Read the model definition and answer for the solid it produces. Units are mm, in the model's axes. A direction names the side the tool comes from. Round coordinates to 2 decimals unless told otherwise and drop trailing zeros. Order: outer loops, then holes, each group sorted by start corner. A loop starts at its lowest first (then second) coordinate and runs counter-clockwise, first axis right, second up. Notation, with made-up numbers: M 87.25,-17 L 119.25,-17 A23 ccw 119.25,14 Z; hole C 24,46 d3. An arc over 180 degrees is marked long. Answer as CSV lines item,"result".
```python
from build123d import *

# Parameters (mm, degrees)
SKETCH004_W     = 40
SKETCH004_H     = 40
PAD001_DEPTH    = 40
SKETCH005_W     = 38.216385
SKETCH005_H     = 40.583008
POCKET002_DEPTH = 11.7
SKETCH006_R     = 1.75
POCKET003_DEPTH = 40.001
SKETCH007_W     = 20
SKETCH007_H     = 28
POCKET004_DEPTH = 35
SKETCH009_R     = 11
POCKET005_DEPTH = 28
SKETCH011_R     = 2.75
POCKET006_DEPTH = 36
SKETCH012_R     = 1.9
POCKET007_DEPTH = 7
CHAMFER003_SIZE = 0.9
SKETCH020_R     = 4.692288
POCKET013_DEPTH = 40.001
FILLET_R        = 3
SKETCH021_W     = 5
SKETCH021_H     = 10
POCKET014_DEPTH = 9
SKETCH022_W     = 5
SKETCH022_H     = 10
POCKET015_DEPTH = 12
SKETCH023_W     = 20
SKETCH023_H     = 14.49538
POCKET016_DEPTH = 20
CHAMFER006_SIZE = 3
CHAMFER007_SIZE = 2
FILLET001_R     = 1


with BuildPart() as part:
    # Sketch004 → Pad001 (new body)
    with BuildSketch(Plane.XY):
        Rectangle(SKETCH004_W, SKETCH004_H)
    extrude(amount=PAD001_DEPTH)

    # Sketch005 (on Face5 of Pad001) → Pocket002 (cut)
    with BuildSketch(Plane(origin=(0, 0, 0), x_dir=(1, 0, 0), z_dir=(0, 0, -1))):
        with Locations((-19.108192, -20.291504)):
            Rectangle(SKETCH005_W, SKETCH005_H)
    extrude(amount=-POCKET002_DEPTH, mode=Mode.SUBTRACT)

    # Sketch006 (on Face4 of Pocket002) → Pocket003 (cut, through all)
    with BuildSketch(Plane(origin=(0, 0, 0), x_dir=(1, 0, 0), z_dir=(0, 0, -1))):
        with Locations((-15.5, 15.5)):
            Circle(SKETCH006_R)
        with Locations((15.5, 15.5)):
            Circle(SKETCH006_R)
        with Locations((-15.5, -15.5)):
            Circle(SKETCH006_R)
        with Locations((15.5, -15.5)):
            Circle(SKETCH006_R)
    extrude(amount=-POCKET003_DEPTH, mode=Mode.SUBTRACT)

    # Sketch007 (on Face1 of Pocket003) → Pocket004 (cut)
    with BuildSketch(Plane(origin=(0, 20, 0), x_dir=(-1, 0, 0), z_dir=(0, 1, 0))):
        with Locations((0, 24)):
            Rectangle(SKETCH007_W, SKETCH007_H)
    extrude(amount=-POCKET004_DEPTH, mode=Mode.SUBTRACT)

    # Sketch009 (on Face9 of Pocket004) → Pocket005 (cut)
    with BuildSketch(Plane.XY.offset(40)):
        Circle(SKETCH009_R)
    extrude(amount=-POCKET005_DEPTH, mode=Mode.SUBTRACT)

    # Sketch011 (on Face9 of Pocket005) → Pocket006 (cut)
    with BuildSketch(Plane.XY.offset(40)):
        with Locations((-15.5, -15.5)):
            Circle(SKETCH011_R)
        with Locations((-15.5, 15.5)):
            Circle(SKETCH011_R)
        with Locations((15.5, 15.5)):
            Circle(SKETCH011_R)
        with Locations((15.5, -15.5)):
            Circle(SKETCH011_R)
    extrude(amount=-POCKET006_DEPTH, mode=Mode.SUBTRACT)

    # Sketch012 (on Face9 of Pocket006) → Pocket007 (cut)
    with BuildSketch(Plane.XY.offset(40)):
        with Locations((0, 15.5)):
            Circle(SKETCH012_R)
        with Locations((15.5, 0)):
            Circle(SKETCH012_R)
        with Locations((0, -15.5)):
            Circle(SKETCH012_R)
        with Locations((-15.5, 0)):
            Circle(SKETCH012_R)
    extrude(amount=-POCKET007_DEPTH, mode=Mode.SUBTRACT)

    # Chamfer003
    chamfer003_edges = [part.edges().sort_by_distance(p)[0] for p in [
        (10.747093, 2.345208, 12),
        (0, -11, 38),
        (10.747093, -2.345208, 12),
    ]]
    chamfer(chamfer003_edges, length=CHAMFER003_SIZE)

    # Sketch020 (on Face19 of Chamfer003) → Pocket013 (cut, through all)
    with BuildSketch(Plane(origin=(0, 0, 0), x_dir=(1, 0, 0), z_dir=(0, 0, -1))):
        Circle(SKETCH020_R)
    extrude(amount=-POCKET013_DEPTH, mode=Mode.SUBTRACT)

    # Fillet
    fillet_edges = [part.edges().sort_by_distance(p)[0] for p in [
        (-4.692288, 0, 5),
        (0, 4.692288, 5),
    ]]
    fillet(fillet_edges, radius=FILLET_R)

    # Sketch021 (on Face22 of Fillet) → Pocket014 (cut)
    with BuildSketch(Plane.YZ.offset(20)):
        with Locations((0, 31)):
            Rectangle(SKETCH021_W, SKETCH021_H)
    extrude(amount=-POCKET014_DEPTH, mode=Mode.SUBTRACT)

    # Sketch022 → Pocket015 (cut)
    with BuildSketch(Plane.XZ.offset(20)):
        with Locations((0, 31)):
            Rectangle(SKETCH022_W, SKETCH022_H)
    extrude(amount=-POCKET015_DEPTH, mode=Mode.SUBTRACT)

    # Sketch023 (on Face13 of Pocket015) → Pocket016 (cut)
    with BuildSketch(Plane(origin=(-20, 0, 0), x_dir=(0, -1, 0), z_dir=(-1, 0, 0))):
        with Locations((0, 40.24769)):
            Rectangle(SKETCH023_W, SKETCH023_H)
    extrude(amount=-POCKET016_DEPTH, mode=Mode.SUBTRACT)

    # Chamfer006
    chamfer006_edges = [part.edges().sort_by_distance(p)[0] for p in [
        (0, -20, 26),
        (20, 0, 26),
    ]]
    chamfer(chamfer006_edges, length=CHAMFER006_SIZE)

    # Chamfer007
    chamfer007_edges = [part.edges().sort_by_distance(p)[0] for p in [
        (-20, -20, 20),
        (-20, 20, 25.85),
        (20, -20, 20),
        (20, 20, 20),
    ]]
    chamfer(chamfer007_edges, length=CHAMFER007_SIZE)

    # Fillet001
    fillet001_edges = [part.edges().sort_by_distance(p)[0] for p in [
        (-2.5, -20, 31),
        (2.5, -20, 31),
        (20, -2.5, 31),
        (20, 2.5, 31),
    ]]
    fillet(fillet001_edges, radius=FILLET001_R)


solid = part.part
```
Item 1: A tool of negligible diameter and unlimited length cuts with its end or side. For faces 4 (the face through (0, -15, 24)), 5 (the face through (-5.41, -0.51, 4.93)), 6 (the face through (-15, 0, 33)), 7 (the face through (15, 2.5, 31)), 8 (the face through (15.142, 18.227, 22.252)), from which of +Z, -Z, +X, -X, +Y, -Y can it reach the whole face along a straight path? Write none if from no direction.
Ans:
face 4,"+Y"
face 5,"+Z, -Z, +Y"
face 6,"+Z, -X"
face 7,"+X"
face 8,"+Z"
Item 2: Find the intervals of material crossed by probe 1 along Z at (x, y) = (3, -12); probe 2 along X at (y, z) = (-11, 28.5); probe 3 along Y at (x, z) = (15.5, 32), in increasing order. Write a range as [from, to].
Ans:
probe 1,"[0, 10], [38, 40]"
probe 2,"[-20, -10], [10, 20]"
probe 3,"[-20, -18.25], [-12.75, -2.5], [2.5, 12.75], [18.25, 20]"
Item 3: A cutting plane is placed at C-C, the plane y = 15.5. Determine the outline of the cut face in (x, z).
Ans:
outline,"M -20,11.7 L -18.25,11.7 L -18.25,40 L -20,40 Z; M -12.75,11.7 L -10,11.7 L -10,38 L -1.9,38 L -1.9,40 L -12.75,40 Z; M 0,0 L 13.75,0 L 13.75,4 L 12.75,4 L 12.75,40 L 1.9,40 L 1.9,38 L 10,38 L 10,10 L 0,10 Z; M 17.25,0 L 20,0 L 20,40 L 18.25,40 L 18.25,4 L 17.25,4 Z"
Item 4: A cutting plane is placed at D-D, the plane z = 14. Determine the outline of the cut face in (x, y), and give its area (3 significant figures).
Ans:
outline,"M -20,-18 L -18,-20 L 18,-20 L 20,-18 L 20,18 L 18,20 L 10,20 L 10,4.58 A11 cw 10,-4.58 L 10,-15 L -10,-15 L -10,-4.58 A11 cw -10,4.58 L -10,20 L -18,20 L -20,18 Z; hole C -15.5,-15.5 d5.5; hole C -15.5,15.5 d5.5; hole C 15.5,-15.5 d5.5; hole C 15.5,15.5 d5.5"
area,"785 mm2"
Item 5: A cutting plane is placed at B-B, the plane x = -15.5. Determine the outline of the cut face in (y, z), and give its area (3 significant figures).
Ans:
outline,"M -20,0 L -17.25,0 L -17.25,4 L -18.25,4 L -18.25,40 L -20,40 Z; M -13.75,0 L 0,0 L 0,11.7 L 12.75,11.7 L 12.75,40 L 10,40 L 10,33 L -10,33 L -10,40 L -12.75,40 L -12.75,4 L -13.75,4 Z; M 18.25,11.7 L 20,11.7 L 20,40 L 18.25,40 Z"
area,"858 mm2"
Item 6: Flat-ended cylindrical pins translate along their axes: pin 1 (2.5 mm diameter, centred on x = 15.5, y = 0, fed in from +Z); pin 2 (2.5 mm diameter, centred on x = 0, y = 15.5, fed in from +Z). Find the tip coordinate at first contact, or state that the pin passes through.
Ans:
pin 1,"z = 26"
pin 2,"z = 10"
Item 7: Determine the mould class of faces 1 (the face through (-17, -14, 4)), 2 (the face through (14, 0, 26)), 3 (the face through (12.753, -15.379, 22.252)) for opening direction Z: +Z half, -Z half, draft (parallel to the pull), parting line (faces both ways), or undercut.
Ans:
face 1,"+Z half"
face 2,"undercut"
face 3,"draft"
